Part model, mm, in its own coordinate system. Face numbers are marked on the shaded views. Give positions to 0.01 mm unless a question says otherwise; leave off trailing zeros. Order: outer loops, then holes, each group sorted by start corner. A loop starts at its lowest first (then second) coordinate and runs counter-clockwise, first axis right, second up. Notation, with made-up numbers: (18, 48) - (29, 48) arc R30 cw to (29, 85) - close; hole circle Ø9 at (47, 70). An arc over 180 degrees is marked (long way). One line per item, written item: value.
Autodesk Inventor part; units mm, degrees
ref_plane "Work Plane1" through (1.525, 0, 0) normal (0, 0, 1) x (1, 0, 0)
ref_plane "YZ Plane" through (0, 0, 0) normal (1, 0, 0) x (0, 1, 0)
ref_plane "XZ Plane" through (0, 0, 0) normal (0, 1, 0) x (-1, 0, 0)
sketch "Szkic1" plane through (0, 0, 0) normal (0, 0, 1) x (1, 0, 0)
  line L0 (0, 3.6) -> (0, 2.5)
  line L1 (12, 2.5) -> (28, 2.5)
  line L2 (28, 2.5) -> (28, 0)
  line L3 (28, 0) -> (-0.2001, 0)
  line L4 (-5.8401, 0) -> (33.64, 0)
  line L5 (-0.2001, 0) -> (-0.2001, 3.6)
  line L6 (-0.2001, 3.6) -> (0, 3.6)
  line L7 (12, 2.5) -> (11.5091, 2.5)
  line L8 (11.5091, 2.5) -> (0, 2.5)
  line L9 (0, -0.72) -> (0, 4.32)
  dimension "d0" = 28
  dimension "d1" = 16
  dimension "d2" = 5
  dimension "d9" = 0.2001
  dimension "d10" = 7.2
  dimension "d13" = 0.4909
  dimension "d14" = 5
revolve "Bryła" add sketch "Szkic1" angle 360 about axis through (28, 0, 0) along (-1, 0, 0)
sketch "Szkic2" plane through (-0.2001, 0, 0) normal (-1, 0, 0) x (0, 0, 1)
  line L0 (0, 4.6188) -> (4, 2.3094)
  line L1 (4, 2.3094) -> (4, -2.3094)
  line L2 (4, -2.3094) -> (0, -4.6188)
  line L3 (0, -4.6188) -> (-4, -2.3094)
  line L4 (-4, -2.3094) -> (-4, 2.3094)
  line L5 (-4, 2.3094) -> (0, 4.6188)
  point P0 (0, 0)
  point P1 (0, 0)
  dimension "d11" = 8
extrude "Głowica" add sketch "Szkic2" along normal blind 3.45
sketch "Szkic4" plane through (0, 0, 0) normal (0, 0, 1) x (1, 0, 0)
  line L0 (-3.6501, 4) -> (-3.6501, 4.6188)
  line L1 (-3.6501, 4.6188) -> (-3.2928, 4.6188)
  line L2 (-3.2928, 4.6188) -> (-3.6501, 4)
  line L3 (-4.3401, 0) -> (0.4899, 0)
  line L4 (-0.2001, 4.6188) -> (-3.6501, 4.6188)
  line L5 (-3.6501, 2.3094) -> (-3.6501, 4.6188)
  dimension "d5" = 30
  dimension "d19" = 8
revolve "Faza1" cut sketch "Szkic4" angle 360 about axis through (-10, 0, 0) along (1, 0, 0)
thread "Gwint"
chamfer "Faza2" distance 0.4908 distance2 0.4909 1 edges at (28, -2.5, 0) measured on face at (28, 0.9945, -0.5526)
ref_plane "Work Plane1" through (1.525, 0, 0) normal (0, 0, 1) x (1, 0, 0)
equation "\"d0\" = NLG"
equation "\"d1\" = GEL"
equation "\"d2\" = GD"
equation "\"d10\" = SD2"
equation "\"d14\" = BDM"
equation "\"d11\" = SW"
equation "\"d3\" = KOH - SD"
equation "\"d5\" = ANG1"
equation "\"d19\" = SW0"
equation "\"d15\" = GEL"
equation "\"d6\" = -0.5 * SPD + 0.5 * GD"
equation "\"NLG\" = 28"
equation "\"GD\" = NND"
equation "\"BDM\" = NND"
equation "\"KOH\" = 3.65"
equation "\"GEL\" = 16"
equation "\"SW\" = 8"
equation "\"SW0\" = 8"
equation "\"SPD\" = NND - 1.2269 * PTC"
equation "\"SD2\" = 0.9 * SW"
equation "\"SD\" = 0.2"
equation "\"ANG1\" = 30deg"
equation "\"GAL\" = 0.61345 * PTC"
equation "\"GUL\" = 0.61345 * PTC"
equation "\"RR\" = 0.35"
equation "\"GD1\" = THREADDIA - 1.2269 * PTC"
equation "\"THREADDIA\" = 5"
equation "\"SDH\" = 7.55"
equation "\"TOA\" = 30deg"
equation "\"PTC\" = 0.8"
equation "\"NND\" = 5"
equation "\"E0\" = 1.155 * SW"
properties part number "BS 3692 - M5 x 28" material "Stal, miękka"
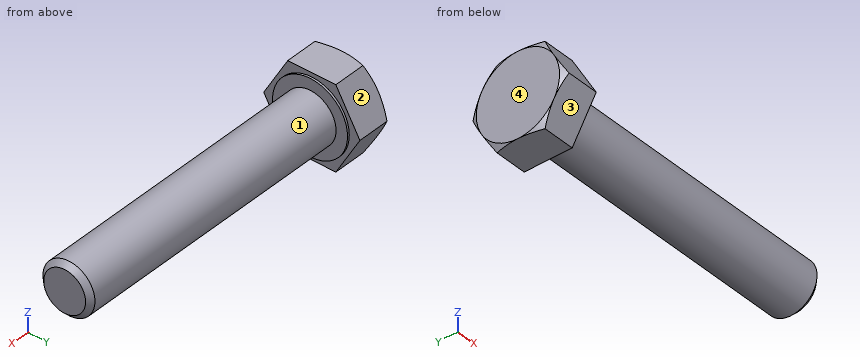
1) Mould opens along Z. For the marked faces 1, 2, 3 and 4 say: released by +Z, released by -Z, zero draft, split by the parting line, or undercut.
Outcome:
face 1: split by the parting line
face 2: released by +Z
face 3: released by -Z
face 4: zero draft
2) Pin check, flat tips, straight feed: pin 1 (1 mm diameter, centred on x = 9.5, z = 2.5, fed in from -Y); pin 2 (4 mm diameter, centred on x = 19.5, y = 1.5, fed in from +Z); pin 3 (3 mm diameter, centred on x = 10.5, y = 2, fed in from -Z). Stop position of each tip, or through.
Outcome:
pin 1: stops at y = -1.5
pin 2: stops at z = 2.5
pin 3: stops at z = -2.45
3) Drill centre lines: line 1 along X through (y, z) = (-2.75, -2.75); line 2 along Z through (x, y) = (12.5, 1.5). Where is each one in solid material? Low to high. Write a range as from..to.
Outcome:
line 1: x = -3.65..-0.2
line 2: z = -2..2
4) Cut at A-A, the plane x = 12.5. Give the cut face in (y, z).
Outcome:
outline: circle Ø5 at (0, 0)
